Can you work these out from the model? Positions are in its coordinate system, mm. A direction names the side the tool comes from. Give positions to 0.01 mm unless a question says otherwise; leave off trailing zeros. Write each loop counter-clockwise with the first axis right and the second up, starting at its lowest first coordinate (ties: lowest second). Pieces come first, ordered by that corner, then holes.
from build123d import *

# Parameters (mm, degrees)
PAD_DEPTH        = 2
SKETCH001_R      = 32
PAD001_DEPTH     = 4
SKETCH002_W      = 28.77499
SKETCH002_H      = 10
PAD002_DEPTH     = 15
HOLE_D           = 5.5
HOLE_DEPTH       = 25
HOLE_CBORE_D     = 10.1
HOLE_CBORE_DEPTH = 4.1


with BuildPart() as part:
    # Sketch → Pad (new body)
    with BuildSketch(Plane.XY):
        with BuildLine():
            ThreePointArc((14.387495, -33), (0, 36), (-14.387495, -33))
            Line((-14.387495, -33), (-14.387495, -43))
            Line((-14.387495, -43), (14.387495, -43))
            Line((14.387495, -43), (14.387495, -33))
        make_face()
    extrude(amount=PAD_DEPTH)

    # Sketch001 (on Face6 of Pad) → Pad001 (join)
    with BuildSketch(Plane.XY.offset(2)):
        with BuildLine():
            ThreePointArc((14.387495, -33), (0, 36), (-14.387495, -33))
            Line((-14.387495, -33), (-14.387495, -43))
            Line((-14.387495, -43), (14.387495, -43))
            Line((14.387495, -43), (14.387495, -33))
        make_face()
        Circle(SKETCH001_R, mode=Mode.SUBTRACT)
    extrude(amount=PAD001_DEPTH)

    # Sketch002 (on Face9 of Pad001) → Pad002 (join)
    with BuildSketch(Plane.XY.offset(6)):
        with Locations((0, -38)):
            Rectangle(SKETCH002_W, SKETCH002_H)
    extrude(amount=PAD002_DEPTH)

    # Hole
    with Locations(Plane(origin=(0, -33, 0), x_dir=(-1, 0, 0), z_dir=(0, 1, 0))):
        with Locations((0, 13.5)):
            CounterBoreHole(HOLE_D / 2, HOLE_CBORE_D / 2, HOLE_CBORE_DEPTH, depth=HOLE_DEPTH)


solid = part.part
(1) Imagine slicing it at D-D, the plane x = 10. Write out the boundary of the cut face in (y, z), plus the area to 3 significant figures.
Returned:
outline: (-43, 0) - (34.58, 0) - (34.58, 6) - (30.4, 6) - (30.4, 2) - (-30.4, 2) - (-30.4, 6) - (-33, 6) - (-33, 21) - (-43, 21) - close
area: 372 mm2
(2) Imagine slicing it at A-A, the plane x = 0. Write out the boundary of the cut face in (y, z).
Returned:
outline: (-43, 0) - (36, 0) - (36, 6) - (32, 6) - (32, 2) - (-32, 2) - (-32, 6) - (-33, 6) - (-33, 8.45) - (-37.1, 8.45) - (-37.1, 10.75) - (-43, 10.75) - close; (-43, 16.25) - (-37.1, 16.25) - (-37.1, 18.55) - (-33, 18.55) - (-33, 21) - (-43, 21) - close
(3) For faces 1 (the face through (-0.2, 32.3, 6)), 2 (the face through (-6.94, -31.24, 3.97)), 3 (the face through (-14.387, -38, 10)), 4 (the face through (-0.358, -40.091, 16.227)), 5 (the face through (0.7, -35, 18.5)), which set-ups out of +Z, -Z, +X, -X, +Y, -Y let a thin tool reach every point of the face, with its end or its side?
Returned:
face 1: +Z, +X, -X, +Y
face 2: +Z
face 3: +Z, -Z, -X, -Y
face 4: +Y, -Y
face 5: +Y
(4) Will these pins go through, and if not, where does the flat tip stop? P1, Ø3, axis at y = -36.5, z = 12.5, coming from the +X side; P2, Ø5, axis at x = -4, z = 15, coming from the +Y side; P3, Ø3, axis at y = -38, z = 6.5, coming from the -X side; P4, Ø3, axis at x = 16.5, y = -16.5, coming from the -Z side.
Returned:
P1: stops at x = 14.39
P2: stops at y = -33
P3: stops at x = -14.39
P4: stops at z = 0
(5) Imagine slicing it at B-B, the plane z = 13.5. Write out the boundary of the cut face in (x, y).
Returned:
outline: (-14.39, -43) - (-2.75, -43) - (-2.75, -37.1) - (-5.05, -37.1) - (-5.05, -33) - (-14.39, -33) - close; (2.75, -43) - (14.39, -43) - (14.39, -33) - (5.05, -33) - (5.05, -37.1) - (2.75, -37.1) - close
(6) If we mould it in two halves opening along X, with no side actions, what happens to faces 6 (the face through (0, 0, 2)), 7 (the face through (14.387, -38, 10)), 8 (the face through (-1, -3, 0))? For each: +X half, -X half, draft (parallel to the pull), parting line (faces both ways), or undercut.
Returned:
face 6: undercut
face 7: +X half
face 8: draft
(7) Imagine slicing it at C-C, the plane y = 0. Write out the boundary of the cut face in (x, z), plus the area to 3 significant figures.
Returned:
outline: (-36, 0) - (36, 0) - (36, 6) - (32, 6) - (32, 2) - (-32, 2) - (-32, 6) - (-36, 6) - close
area: 176 mm2
(8) If I drill on L1, parallel to Z at x = 0, y = -39; L2, parallel to Z at x = 0, y = -36.3; L3, parallel to Z at x = 8, y = 19, over which ranges is the centre line in solid material (lowest first)?
Returned:
L1: z = 0 to 10.75, 16.25 to 21
L2: z = 0 to 8.45, 18.55 to 21
L3: z = 0 to 2
